For this review, take the finished solid that the model builds, in its own axes (mm). A direction names the side the tool comes from. Round coordinates to 2 decimals unless told otherwise and drop trailing zeros. Order: outer loops, then holes, each group sorted by start corner. A loop starts at its lowest first (then second) coordinate and runs counter-clockwise, first axis right, second up. Notation, with made-up numbers: (-6, -23) -> (24, -23) arc R31 ccw to (24, 13) -> close; hole circle Ø8 at (81.25, -20.5). An arc over 180 degrees is marked (long way). Use a Markdown table: item, result. Add a question column.
1) Wall thickness on line 1 along Y through (x, z) = (0, -1.7); line 2 along X through (y, z) = (0.5, -1.25); line 3 along Y through (x, z) = (2.5, 0): over which ranges is each line inside the solid? List them lowest first. Write a range as [from, to].
2) Consider section A-A (x = 0). State the section outline as (y, z) points, plus the area to 3 significant figures.
3) Consider section C-C (z = 4). State the section outline as (x, y) points.
4) Consider section D-D (z = -4). State the section outline as (x, y) points, plus the area to 3 significant figures.
5) Machinability: for faces 5 (the face through (-4.3, -7.1, 5.5)), 6 (the face through (-1.756, -7.907, 2.542)), which of the approach directions +Z, -Z, +X, -X, +Y, -Y give a long, thin tool a straight path to every point of the face, cutting with its end or side? Answer none if there is none.
6) Clearance check with flat-ended pins moving along their axes: P1, Ø13, axis at x = 0, y = 0, coming from the +Z side; P2, Ø13, axis at x = -2.5, y = -2, coming from the +Z side; P3, Ø2, axis at x = -3.5, z = 4, coming from the -Y side; P4, Ø5, axis at y = 5, z = -1, coming from the +X side. State where each tip first meets the part, or that it passes through.
7) Draft analysis for pull direction Y (two halves, no side actions). For faces 1 (the face through (3.233, -1.341, -2.965)), 2 (the face through (4, 0, -5.5)), 3 (the face through (-2.1, -9.46, 5.32)), 4 (the face through (3.5, -1.7, -0.5)), state which applies: pulls with the +Y half, pulls with the -Y half, needs draft (parallel to the pull), parting line crosses it, or undercut.
```python
from build123d import *

# Parameters (mm, degrees)
F0_R          = 11
F1_DEPTH      = 5.5
F1_DEPTH_BACK = 5.5
F3_SIZE2      = 2.8
F3_SIZE       = 1.4
F4_SIZE2      = 1.4
F4_SIZE       = 2.8
F5_R          = 8.1
F6_DEPTH      = 6
F7_R          = 3.5
F8_DEPTH      = 5


with BuildPart() as f1:
    # F0 (on Top) → F1 (new body, two sides)
    with BuildSketch(Plane.XY) as f1_sk:
        Circle(F0_R)
    extrude(amount=F1_DEPTH)
    extrude(f1_sk.sketch, amount=-F1_DEPTH_BACK)

    # F3
    f3_edges = [f1.edges().sort_by_distance(p)[0] for p in [
        (-11, 0, 5.5),
    ]]
    f3_side = f1.faces().sort_by_distance((0, 0, 5.5))[0]
    chamfer(f3_edges, length=F3_SIZE, length2=F3_SIZE2, reference=f3_side)

    # F4
    f4_edges = [f1.edges().sort_by_distance(p)[0] for p in [
        (-11, 0, -5.5),
    ]]
    f4_side = f1.faces().sort_by_distance((-11, 0, -2.75))[0]
    chamfer(f4_edges, length=F4_SIZE, length2=F4_SIZE2, reference=f4_side)

    # F5 (on face) → F6 (cut)
    with BuildSketch(Plane.XY.offset(5.5)):
        Circle(F5_R)
    extrude(amount=-F6_DEPTH, mode=Mode.SUBTRACT)

    # F7 (on face) → F8 (cut, through all)
    with BuildSketch(Plane.XY.offset(-0.5)):
        Circle(F7_R)
    extrude(amount=-F8_DEPTH, mode=Mode.SUBTRACT)


solid = f1.part
```
Results list:
| question | item | result |
|---|---|---|
| 1 | line 1 | [-11, -3.5], [3.5, 11] |
| 1 | line 2 | [-10.99, -3.46], [3.46, 10.99] |
| 1 | line 3 | [-10.71, -7.7], [7.7, 10.71] |
| 2 | outline | (-11, -2.7) -> (-9.6, -5.5) -> (-3.5, -5.5) -> (-3.5, -0.5) -> (-8.1, -0.5) -> (-8.1, 5.5) -> (-9.6, 5.5) -> (-11, 2.7) -> close; (3.5, -5.5) -> (9.6, -5.5) -> (11, -2.7) -> (11, 2.7) -> (9.6, 5.5) -> (8.1, 5.5) -> (8.1, -0.5) -> (3.5, -0.5) -> close |
| 2 | area | 102 mm2 |
| 3 | outline | circle Ø20.7 at (0, 0); hole circle Ø16.2 at (0, 0) |
| 4 | outline | circle Ø20.7 at (0, 0); hole circle Ø7 at (0, 0) |
| 4 | area | 298 mm2 |
| 5 | face 5 | +Z, +X, -X, +Y, -Y |
| 5 | face 6 | +Z |
| 6 | P1 | z = -0.5 |
| 6 | P2 | z = 5.5 |
| 6 | P3 | y = -10.36 |
| 6 | P4 | x = 10.71 |
| 7 | face 1 | undercut |
| 7 | face 2 | needs draft |
| 7 | face 3 | parting line crosses it |
| 7 | face 4 | undercut |
